For this review, take the finished solid that the model builds, in its own axes (mm). A direction names the side the tool comes from. Give positions to 0.01 mm unless a question says otherwise; leave off trailing zeros. Loops run counter-clockwise (first coordinate to the right, second up) from the corner with the lowest first, then second, coordinate; pieces in that order, holes last. Notation, with made-up numbers: (29, 18) - (72, 18) arc R29 ccw to (72, 55) - close; hole circle Ø4 at (88, 25.5). An arc over 180 degrees is marked (long way). Answer in a Markdown table with one row per item.
```python
from build123d import *

# Parameters (mm, degrees)
BOSS_EXTRUDE1_DEPTH = 200
FILLET1_R           = 10
SKETCH2_W           = 39
SKETCH2_H           = 59.5
CUT_EXTRUDE1_DEPTH  = 2
SKETCH3_W           = 71.2
SKETCH3_H           = 26.2
CUT_EXTRUDE2_DEPTH  = 10
CUT_EXTRUDE4_DEPTH  = 215
SKETCH10_R          = 0.3
CUT_EXTRUDE5_DEPTH  = 10


with BuildPart() as part:
    # Sketch1 → Boss-Extrude1 (new body)
    with BuildSketch(Plane.XY):
        Polygon((0, 0), (100, 0), (50, 50), (0, 50), align=None)
    extrude(amount=BOSS_EXTRUDE1_DEPTH)

    # Fillet1
    fillet1_edges = [part.edges().sort_by_distance(p)[0] for p in [
        (0, 25, 200),
        (0, 25, 0),
    ]]
    fillet(fillet1_edges, radius=FILLET1_R)

    # Sketch2 → Cut-Extrude1 (cut)
    with BuildSketch(Plane(origin=(50, 50, 0), x_dir=(0, 0, -1), z_dir=(0.707106781, 0.707106781, 0))):
        with Locations((-46.962285567, -35.355339059)):
            Rectangle(SKETCH2_W, SKETCH2_H)
    extrude(amount=-CUT_EXTRUDE1_DEPTH, mode=Mode.SUBTRACT)

    # Sketch3 → Cut-Extrude2 (cut)
    with BuildSketch(Plane(origin=(50, 50, 0), x_dir=(0, 0, -1), z_dir=(0.707106781, 0.707106781, 0))):
        with Locations((-146.711084233, -35.355339059)):
            Rectangle(SKETCH3_W, SKETCH3_H)
    extrude(amount=-CUT_EXTRUDE2_DEPTH, mode=Mode.SUBTRACT)

    # Sketch6 → Cut-Extrude4 (cut)
    with BuildSketch(Plane.XY.offset(200)):
        Polygon((50, 44), (80.771793261, 6), (16, 6), (16, 44), align=None)
    extrude(amount=-CUT_EXTRUDE4_DEPTH, mode=Mode.SUBTRACT)

    # Sketch10 → Cut-Extrude5 (cut)
    with BuildSketch(Plane(origin=(50, 50, 0), x_dir=(0, 0, -1), z_dir=(0.707106781, 0.707106781, 0))):
        with Locations((-90.936655298, -35.355339059)):
            Circle(SKETCH10_R)
        with Locations((-85.936655298, -35.355339059)):
            Circle(SKETCH10_R)
    extrude(amount=-CUT_EXTRUDE5_DEPTH, mode=Mode.SUBTRACT)


solid = part.part
```
1. We need section C-C, the plane z = 172.5. Give the boundary of the cut face in (x, y).
Values:
| item | result |
|---|---|
| outline | (0, 0) - (100, 0) - (84.26, 15.74) - (77.98, 9.45) - (80.77, 6) - (16, 6) - (16, 44) - (50, 44) - (61.4, 29.92) - (65.74, 34.26) - (50, 50) - (0, 50) - close |
2. Wall thickness on line 1 (Z direction, x = 74, y = 25); line 2 (Y direction, x = 27, z = 51); line 3 (X direction, y = 28, z = 90.5): over which ranges is each line inside the solid? List them lowest first. Write a range as [from, to].
Values:
| item | result |
|---|---|
| line 1 | z = [0, 27.46], [66.46, 111.11], [182.31, 200] |
| line 2 | y = [0, 6], [44, 50] |
| line 3 | x = [0, 16], [62.96, 72] |
3. We need section A-A, the plane x = 26. Give the boundary of the cut face in (y, z).
Values:
| item | result |
|---|---|
| outline | (0, 0) - (6, 0) - (6, 200) - (0, 200) - close; (44, 0) - (50, 0) - (50, 200) - (44, 200) - close |
4. For faces 5 (the face through (49, 6, 101)), 6 (the face through (25, 50, 99)), 7 (the face through (63.598, 32.124, 147.209)), list the 3-axis set-ups (+Z, -Z, +X, -X, +Y, -Y) from which the entire face can be reached by the end or side of a thin tool; tool diameter is ignored.
Values:
| item | result |
|---|---|
| face 5 | +Z, -Z |
| face 6 | +Z, -Z, +X, -X, +Y |
| face 7 | +X |
5. We need section D-D, the plane y = 42. Give the boundary of the cut face in (x, z).
Values:
| item | result |
|---|---|
| outline | (0, 10) arc R10 ccw to (10, 0) - (16, 0) - (16, 200) - (10, 200) arc R10 ccw to (0, 190) - close; (51.62, 0) - (58, 0) - (58, 27.46) - (55.17, 27.46) - (55.17, 66.46) - (58, 66.46) - (58, 200) - (51.62, 200) - close |
6. Mouldability with a two-part tool opening along Z and no side actions: class faces 1 (the face through (2.85, 24.65, 196.99)), 2 (the face through (72.224, 22.511, 91.158)), 3 (the face through (75, 24, 27.462)), 4 (the face through (48, 5, 0)) as released by +Z, released by -Z, zero draft, split by the parting line, or undercut.
Values:
| item | result |
|---|---|
| face 1 | released by +Z |
| face 2 | undercut |
| face 3 | undercut |
| face 4 | released by -Z |
7. Clearance check with flat-ended pins moving along their axes: pin 1 (4 mm diameter, centred on x = 55.5, z = 79.5, fed in from +Y); pin 2 (2 mm diameter, centred on y = 5, z = 37, fed in from +X); pin 3 (8 mm diameter, centred on y = 16.5, z = 123.5, fed in from +X). State where each tip first meets the part, or that it passes through.
Values:
| item | result |
|---|---|
| pin 1 | stops at y = 46.5 |
| pin 2 | stops at x = 93.17 |
| pin 3 | stops at x = 87.5 |
8. We need section B-B, the plane z = 104. Give the boundary of the cut face in (x, y), and give its area (3 significant figures).
Values:
| item | result |
|---|---|
| outline | (0, 0) - (100, 0) - (50, 50) - (0, 50) - close; hole (16, 6) - (80.77, 6) - (50, 44) - (16, 44) - close |
| area | 1,870 mm^2 |
